Design review of the part built by this model. Coordinates are the model's own, in mm. Face numbers are marked on the shaded views. A direction names the side the tool comes from. Give positions to 0.01 mm unless a question says otherwise; leave off trailing zeros. Write each loop counter-clockwise with the first axis right and the second up, starting at its lowest first coordinate (ties: lowest second). Pieces come first, ordered by that corner, then holes. Notation, with made-up numbers: (54.25, 68) -> (80.25, 68) arc R15 ccw to (80.25, 91) -> close; hole circle Ø3 at (37, 14.25). An arc over 180 degrees is marked (long way). Return JSON: item names as keys, results as strings. Group by question number.
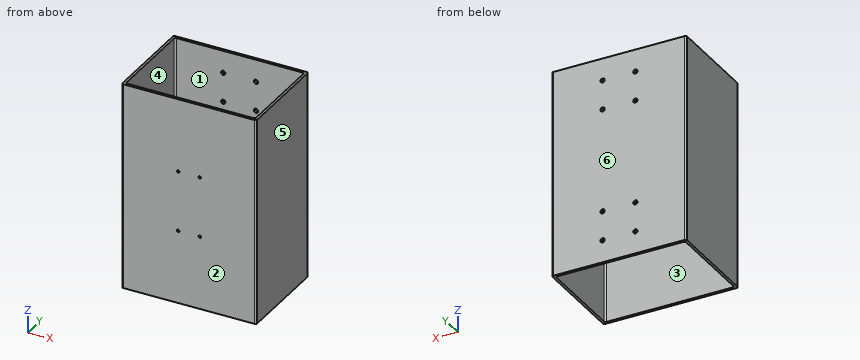
from build123d import *

# Parameters (mm, degrees)
SKETCH1_W                      = 156
SKETCH1_H                      = 111
SKETCH1_W_2                    = 150
SKETCH1_H_2                    = 105
EXTRUDE_THIN1_DEPTH            = 120
FILLET1_R                      = 2
CUT_EXTRUDE1_REACH             = 183.122
SKETCH5_R                      = 2.5
CUT_EXTRUDE1_DIRECTION_2_DEPTH = 182.121506177
CUT_EXTRUDE2_REACH             = 183.122
SKETCH7_R                      = 1.5
CUT_EXTRUDE2_DIRECTION_2_DEPTH = 182.121506177


with BuildPart() as part:
    # Sketch1 → Extrude-Thin1 (new, symmetric)
    with BuildSketch(Plane.XY):
        Rectangle(SKETCH1_W, SKETCH1_H)
        Rectangle(SKETCH1_W_2, SKETCH1_H_2, mode=Mode.SUBTRACT)
    extrude(amount=EXTRUDE_THIN1_DEPTH, both=True)

    # Fillet1
    fillet1_edges = [part.edges().sort_by_distance(p)[0] for p in [
        (-75, 52.5, 0),
        (-75, -52.5, 0),
        (75, -52.5, 0),
        (75, 52.5, 0),
        (-78, 55.5, 0),
        (78, 55.5, 0),
        (78, -55.5, 0),
        (-78, -55.5, 0),
    ]]
    fillet(fillet1_edges, radius=FILLET1_R)

    # Sketch5 → Cut-Extrude1 (cut, up to next)
    with BuildSketch(Plane(origin=(0, 55.5, 0), x_dir=(1, 0, 0), z_dir=(0, 1, 0)), mode=Mode.PRIVATE) as cut_extrude1_sk1:
        with Locations((-19, 60)):
            Circle(SKETCH5_R)
    cut_extrude1_tool1 = extrude(cut_extrude1_sk1.sketch, amount=-CUT_EXTRUDE1_REACH, mode=Mode.PRIVATE) & part.part
    # Sketch5 → Cut-Extrude1 (cut, up to next)
    with BuildSketch(Plane(origin=(0, 55.5, 0), x_dir=(1, 0, 0), z_dir=(0, 1, 0)), mode=Mode.PRIVATE) as cut_extrude1_sk2:
        with Locations((19, 60)):
            Circle(SKETCH5_R)
    cut_extrude1_tool2 = extrude(cut_extrude1_sk2.sketch, amount=-CUT_EXTRUDE1_REACH, mode=Mode.PRIVATE) & part.part
    # Sketch5 → Cut-Extrude1 (cut, up to next)
    with BuildSketch(Plane(origin=(0, 55.5, 0), x_dir=(1, 0, 0), z_dir=(0, 1, 0)), mode=Mode.PRIVATE) as cut_extrude1_sk3:
        with Locations((19, -60)):
            Circle(SKETCH5_R)
    cut_extrude1_tool3 = extrude(cut_extrude1_sk3.sketch, amount=-CUT_EXTRUDE1_REACH, mode=Mode.PRIVATE) & part.part
    # Sketch5 → Cut-Extrude1 (cut, up to next)
    with BuildSketch(Plane(origin=(0, 55.5, 0), x_dir=(1, 0, 0), z_dir=(0, 1, 0)), mode=Mode.PRIVATE) as cut_extrude1_sk4:
        with Locations((-19, -60)):
            Circle(SKETCH5_R)
    cut_extrude1_tool4 = extrude(cut_extrude1_sk4.sketch, amount=-CUT_EXTRUDE1_REACH, mode=Mode.PRIVATE) & part.part
    # Sketch5 → Cut-Extrude1 (cut, up to next)
    with BuildSketch(Plane(origin=(0, 55.5, 0), x_dir=(1, 0, 0), z_dir=(0, 1, 0)), mode=Mode.PRIVATE) as cut_extrude1_sk5:
        with Locations((-19, 94.1)):
            Circle(SKETCH5_R)
    cut_extrude1_tool5 = extrude(cut_extrude1_sk5.sketch, amount=-CUT_EXTRUDE1_REACH, mode=Mode.PRIVATE) & part.part
    # Sketch5 → Cut-Extrude1 (cut, up to next)
    with BuildSketch(Plane(origin=(0, 55.5, 0), x_dir=(1, 0, 0), z_dir=(0, 1, 0)), mode=Mode.PRIVATE) as cut_extrude1_sk6:
        with Locations((19, 94.1)):
            Circle(SKETCH5_R)
    cut_extrude1_tool6 = extrude(cut_extrude1_sk6.sketch, amount=-CUT_EXTRUDE1_REACH, mode=Mode.PRIVATE) & part.part
    # Sketch5 → Cut-Extrude1 (cut, up to next)
    with BuildSketch(Plane(origin=(0, 55.5, 0), x_dir=(1, 0, 0), z_dir=(0, 1, 0)), mode=Mode.PRIVATE) as cut_extrude1_sk7:
        with Locations((19, -94.1)):
            Circle(SKETCH5_R)
    cut_extrude1_tool7 = extrude(cut_extrude1_sk7.sketch, amount=-CUT_EXTRUDE1_REACH, mode=Mode.PRIVATE) & part.part
    # Sketch5 → Cut-Extrude1 (cut, up to next)
    with BuildSketch(Plane(origin=(0, 55.5, 0), x_dir=(1, 0, 0), z_dir=(0, 1, 0)), mode=Mode.PRIVATE) as cut_extrude1_sk8:
        with Locations((-19, -94.1)):
            Circle(SKETCH5_R)
    cut_extrude1_tool8 = extrude(cut_extrude1_sk8.sketch, amount=-CUT_EXTRUDE1_REACH, mode=Mode.PRIVATE) & part.part
    add(cut_extrude1_tool1.solids().sort_by_distance((-19, 55.5, -60))[0], mode=Mode.SUBTRACT)
    add(cut_extrude1_tool2.solids().sort_by_distance((19, 55.5, -60))[0], mode=Mode.SUBTRACT)
    add(cut_extrude1_tool3.solids().sort_by_distance((19, 55.5, 60))[0], mode=Mode.SUBTRACT)
    add(cut_extrude1_tool4.solids().sort_by_distance((-19, 55.5, 60))[0], mode=Mode.SUBTRACT)
    add(cut_extrude1_tool5.solids().sort_by_distance((-19, 55.5, -94.1))[0], mode=Mode.SUBTRACT)
    add(cut_extrude1_tool6.solids().sort_by_distance((19, 55.5, -94.1))[0], mode=Mode.SUBTRACT)
    add(cut_extrude1_tool7.solids().sort_by_distance((19, 55.5, 94.1))[0], mode=Mode.SUBTRACT)
    add(cut_extrude1_tool8.solids().sort_by_distance((-19, 55.5, 94.1))[0], mode=Mode.SUBTRACT)

    # Sketch5 → Cut-Extrude1 direction 2 (cut)
    with BuildSketch(Plane(origin=(0, 55.5, 0), x_dir=(1, 0, 0), z_dir=(0, 1, 0))):
        with Locations((-19, 60)):
            Circle(SKETCH5_R)
        with Locations((19, 60)):
            Circle(SKETCH5_R)
        with Locations((19, -60)):
            Circle(SKETCH5_R)
        with Locations((-19, -60)):
            Circle(SKETCH5_R)
        with Locations((-19, 94.1)):
            Circle(SKETCH5_R)
        with Locations((19, 94.1)):
            Circle(SKETCH5_R)
        with Locations((19, -94.1)):
            Circle(SKETCH5_R)
        with Locations((-19, -94.1)):
            Circle(SKETCH5_R)
    extrude(amount=CUT_EXTRUDE1_DIRECTION_2_DEPTH, mode=Mode.SUBTRACT)

    # Sketch7 → Cut-Extrude2 (cut, up to next)
    with BuildSketch(Plane(origin=(0, -55.5, 0), x_dir=(-1, 0, 0), z_dir=(0, -1, 0)), mode=Mode.PRIVATE) as cut_extrude2_sk1:
        with Locations((-12.475, -34.95)):
            Circle(SKETCH7_R)
    cut_extrude2_tool1 = extrude(cut_extrude2_sk1.sketch, amount=-CUT_EXTRUDE2_REACH, mode=Mode.PRIVATE) & part.part
    # Sketch7 → Cut-Extrude2 (cut, up to next)
    with BuildSketch(Plane(origin=(0, -55.5, 0), x_dir=(-1, 0, 0), z_dir=(0, -1, 0)), mode=Mode.PRIVATE) as cut_extrude2_sk2:
        with Locations((12.475, -34.95)):
            Circle(SKETCH7_R)
    cut_extrude2_tool2 = extrude(cut_extrude2_sk2.sketch, amount=-CUT_EXTRUDE2_REACH, mode=Mode.PRIVATE) & part.part
    # Sketch7 → Cut-Extrude2 (cut, up to next)
    with BuildSketch(Plane(origin=(0, -55.5, 0), x_dir=(-1, 0, 0), z_dir=(0, -1, 0)), mode=Mode.PRIVATE) as cut_extrude2_sk3:
        with Locations((-12.475, 34.95)):
            Circle(SKETCH7_R)
    cut_extrude2_tool3 = extrude(cut_extrude2_sk3.sketch, amount=-CUT_EXTRUDE2_REACH, mode=Mode.PRIVATE) & part.part
    # Sketch7 → Cut-Extrude2 (cut, up to next)
    with BuildSketch(Plane(origin=(0, -55.5, 0), x_dir=(-1, 0, 0), z_dir=(0, -1, 0)), mode=Mode.PRIVATE) as cut_extrude2_sk4:
        with Locations((12.475, 34.95)):
            Circle(SKETCH7_R)
    cut_extrude2_tool4 = extrude(cut_extrude2_sk4.sketch, amount=-CUT_EXTRUDE2_REACH, mode=Mode.PRIVATE) & part.part
    add(cut_extrude2_tool1.solids().sort_by_distance((12.475, -55.5, 34.95))[0], mode=Mode.SUBTRACT)
    add(cut_extrude2_tool2.solids().sort_by_distance((-12.475, -55.5, 34.95))[0], mode=Mode.SUBTRACT)
    add(cut_extrude2_tool3.solids().sort_by_distance((12.475, -55.5, -34.95))[0], mode=Mode.SUBTRACT)
    add(cut_extrude2_tool4.solids().sort_by_distance((-12.475, -55.5, -34.95))[0], mode=Mode.SUBTRACT)

    # Sketch7 → Cut-Extrude2 direction 2 (cut)
    with BuildSketch(Plane(origin=(0, -55.5, 0), x_dir=(-1, 0, 0), z_dir=(0, -1, 0))):
        with Locations((-12.475, -34.95)):
            Circle(SKETCH7_R)
        with Locations((12.475, -34.95)):
            Circle(SKETCH7_R)
        with Locations((-12.475, 34.95)):
            Circle(SKETCH7_R)
        with Locations((12.475, 34.95)):
            Circle(SKETCH7_R)
    extrude(amount=CUT_EXTRUDE2_DIRECTION_2_DEPTH, mode=Mode.SUBTRACT)


solid = part.part
Q1. For L1, parallel to X at y = 53, z = -94; L2, parallel to Y at x = 53, z = -87; L3, parallel to X at y = -54, z = 34, list the stretches that pass through material, from the lowest coordinate up. Write a range as from..to.
Q2. Take a section at A-A, the plane x = 19. Give the boundary of the cut face in (y, z).
Q3. Mouldability with a two-part tool opening along X and no side actions: class the marked faces 3, 4, 5 and 6 as +X half, -X half, draft (parallel to the pull), parting line (faces both ways), or undercut.
Q4. Take a section at B-B, the plane z = 60. Give the boundary of the cut face in (x, y), plus the area to 3 significant figures.
Q5. Tool access review of the marked faces 1 and 2: name each direction out of +Z, -Z, +X, -X, +Y, -Y from which nothing blocks a thin tool from reaching the whole face with its end or side.
Q6. Take a section at C-C, the plane z = 7. Give the boundary of the cut face in (x, y), plus the area to 3 significant figures.
Q7. Take a section at D-D, the plane y = -22. Give the boundary of the cut face in (x, z).
Q8. Insertion check: pin 1 (3 mm diameter, centred on x = -19, z = 60, fed in from +Y); pin 2 (2.5 mm diameter, centred on x = 12.475, z = 34.95, fed in from -Y). Each pin has a flat end and moves straight along its axis. Give the tip position at first contact, or say it passes through.
Final values:
{
 "1": {"L1": "x = -78..-21.5, -16.5..16.5, 21.5..78", "L2": "y = -55.5..-52.5, 52.5..55.5", "L3": "x = -77.94..-13.64, -11.31..11.31, 13.64..77.94"},
 "2": {"outline": "(-55.5, -120) -> (-52.5, -120) -> (-52.5, 120) -> (-55.5, 120) -> close; (52.5, -120) -> (55.5, -120) -> (55.5, -96.6) -> (52.5, -96.6) -> close; (52.5, -91.6) -> (55.5, -91.6) -> (55.5, -62.5) -> (52.5, -62.5) -> close; (52.5, -57.5) -> (55.5, -57.5) -> (55.5, 57.5) -> (52.5, 57.5) -> close; (52.5, 62.5) -> (55.5, 62.5) -> (55.5, 91.6) -> (52.5, 91.6) -> close; (52.5, 96.6) -> (55.5, 96.6) -> (55.5, 120) -> (52.5, 120) -> close"},
 "3": {"face 3": "undercut", "face 4": "undercut", "face 5": "+X half", "face 6": "draft"},
 "4": {"outline": "(-78, -53.5) arc R2 ccw to (-76, -55.5) -> (76, -55.5) arc R2 ccw to (78, -53.5) -> (78, 53.5) arc R2 ccw to (76, 55.5) -> (21.5, 55.5) -> (21.5, 52.5) -> (73, 52.5) arc R2 cw to (75, 50.5) -> (75, -50.5) arc R2 cw to (73, -52.5) -> (-73, -52.5) arc R2 cw to (-75, -50.5) -> (-75, 50.5) arc R2 cw to (-73, 52.5) -> (-21.5, 52.5) -> (-21.5, 55.5) -> (-76, 55.5) arc R2 ccw to (-78, 53.5) -> close; (-16.5, 52.5) -> (16.5, 52.5) -> (16.5, 55.5) -> (-16.5, 55.5) -> close", "area": "1,540 mm²"},
 "5": {"face 1": "+Z, -Z", "face 2": "+Z, -Z, +X, -X, -Y"},
 "6": {"outline": "(-78, -53.5) arc R2 ccw to (-76, -55.5) -> (76, -55.5) arc R2 ccw to (78, -53.5) -> (78, 53.5) arc R2 ccw to (76, 55.5) -> (-76, 55.5) arc R2 ccw to (-78, 53.5) -> close; hole (-75, -50.5) arc R2 ccw to (-73, -52.5) -> (73, -52.5) arc R2 ccw to (75, -50.5) -> (75, 50.5) arc R2 ccw to (73, 52.5) -> (-73, 52.5) arc R2 ccw to (-75, 50.5) -> close", "area": "1,570 mm²"},
 "7": {"outline": "(-78, -120) -> (-75, -120) -> (-75, 120) -> (-78, 120) -> close; (75, -120) -> (78, -120) -> (78, 120) -> (75, 120) -> close"},
 "8": {"pin 1": "stops at y = -52.5", "pin 2": "stops at y = 52.5"}
}
